```python
from build123d import *

# Parameters (mm, degrees)
F0_W     = 30
F0_H     = 30
F1_DEPTH = 60
F2_R     = 6.5
F3_DEPTH = 10
F4_R     = 10
F5_DEPTH = 40


with BuildPart() as f1:
    # F0 (on Front) → F1 (new body, symmetric)
    with BuildSketch(Plane.XZ):
        Rectangle(F0_W, F0_H)
    extrude(amount=F1_DEPTH, both=True)

    # F2 (on face) → F3 (join)
    with BuildSketch(Plane.XZ.offset(60)):
        Circle(F2_R)
    extrude(amount=F3_DEPTH)

    # F4 (on face) → F5 (cut)
    with BuildSketch(Plane(origin=(0, 60, 0), x_dir=(-1, 0, 0), z_dir=(0, 1, 0))):
        with Locations((-0.812379, 0)):
            Circle(F4_R)
    extrude(amount=-F5_DEPTH, mode=Mode.SUBTRACT)


solid = f1.part
```
The listing builds one solid part. Answer for the finished solid, in the listing's coordinates (mm). A direction names the side the tool comes from. Give positions to 0.01 mm unless a question says otherwise; leave off trailing zeros. Order: outer loops, then holes, each group sorted by start corner. A loop starts at its lowest first (then second) coordinate and runs counter-clockwise, first axis right, second up.
1) Consider line 1 along Y through (x, z) = (-10.5, 3.75); line 2 along Y through (x, z) = (4.5, -8). Determine where each line is inside the solid, lowest interval first.
Reported:
line 1: y = -60 to 60
line 2: y = -60 to 20
2) Determine the mould class of faces 4 (the face through (-5.158, -64.93, -3.955)), 5 (the face through (-7, 60, 7)), 6 (the face through (1, 20, 0)) for opening direction X: pulls with the +X half, pulls with the -X half, needs draft (parallel to the pull), parting line crosses it, or undercut.
Reported:
face 4: parting line crosses it
face 5: needs draft
face 6: undercut
3) Given P1, Ø5, axis at x = 2, z = 8.5, coming from the -Y side; P2, Ø6, axis at x = 0.5, z = 0, coming from the +Y side, each flat-ended and moving along its own axis, determine where each tip first touches the part or whether it passes through.
Reported:
P1: stops at y = -70
P2: stops at y = 20
4) Find section B-B on z = -1.75. Write down the section's boundary in (x, y).
Reported:
outline: (-15, -60) - (-6.26, -60) - (-6.26, -70) - (6.26, -70) - (6.26, -60) - (15, -60) - (15, 60) - (10.66, 60) - (10.66, 20) - (-9.03, 20) - (-9.03, 60) - (-15, 60) - close
5) Find section C-C on x = 2.5. Write down the section's boundary in (y, z).
Reported:
outline: (-70, -6) - (-60, -6) - (-60, -15) - (60, -15) - (60, -9.86) - (20, -9.86) - (20, 9.86) - (60, 9.86) - (60, 15) - (-60, 15) - (-60, 6) - (-70, 6) - close
6) For faces 1 (the face through (0, -1, -15)), 2 (the face through (2.98, 40.28, -9.762)), 3 (the face through (-7, -60, 0)), determine the directions among +Z, -Z, +X, -X, +Y, -Y from which every point of the face is accessible in a straight line to the end or side of a thin tool.
Reported:
face 1: -Z, +X, -X, +Y, -Y
face 2: +Y
face 3: -Y
7) Find section A-A on y = 25.5. Write down the section's boundary in (x, z).
Reported:
outline: (-15, -15) - (15, -15) - (15, 15) - (-15, 15) - close; hole circle Ø20 at (0.81, 0)
